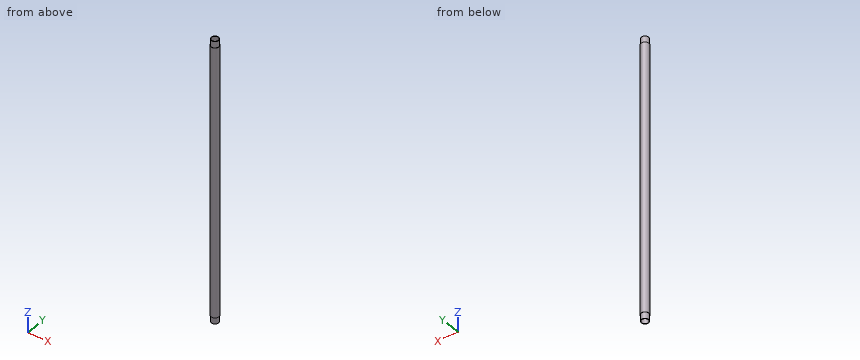
```python
from build123d import *

# Parameters (mm, degrees)
SKETCH2_R           = 6.35
SKETCH2_R_2         = 5.334
BOSS_EXTRUDE1_DEPTH = 457.2


with BuildPart() as part:
    # Sketch2 → Boss-Extrude1 (new body)
    with BuildSketch(Plane.XY):
        Circle(SKETCH2_R)
        Circle(SKETCH2_R_2, mode=Mode.SUBTRACT)
    extrude(amount=BOSS_EXTRUDE1_DEPTH)

    # Sketch3 → Cut-Revolve3 (revolve, cut)
    with BuildSketch(Plane(origin=(0, 0, 0), x_dir=(0, 0, -1), z_dir=(1, 0, 0)), mode=Mode.PRIVATE) as cut_revolve3_sk:
        Polygon((-457.2, 8.954277603), (-457.2, 5.869613211), (-447.050584192, 6.020223087), (-447.050584192, 8.954277603), align=None)
        Polygon((-10.149415808, 8.954277603), (0, 8.954277603), (0, 5.869613211), (-10.149415808, 6.020223087), align=None)
    revolve(cut_revolve3_sk.sketch.rotate(Axis((0, 0, 0), (0, 0, 1)), 90), axis=Axis((0, 0, 0), (0, 0, 1)), mode=Mode.SUBTRACT)


solid = part.part
```
CAD build for the part. Positions are in the model's coordinates, mm. Round coordinates to 2 decimals unless told otherwise and drop trailing zeros. Write each loop counter-clockwise with the first axis right and the second up, starting at its lowest first coordinate (ties: lowest second). Pieces come first, ordered by that corner, then holes.
Item 1: Drop flat-ended pins along their axis: pin 1 Ø6 at (x, z) = (-5, 390.5) entering from -Y; pin 2 Ø2 at (x, z) = (-4.5, 104) entering from -Y; pin 3 Ø6.5 at (x, y) = (-2.5, 0.5) entering from +Z; pin 4 Ø1 at (y, z) = (4.5, 305) entering from +X. Give the stop position or say it passes through.
Filled in:
pin 1: stops at y = -6.03
pin 2: stops at y = -5.3
pin 3: stops at z = 457.2
pin 4: stops at x = 4.93
Item 2: Band-saw the part on A-A on z = 422.5. Write the cut outline in (x, y).
Filled in:
outline: circle Ø12.7 at (0, 0); hole circle Ø10.67 at (0, 0)
Item 3: Drill centre lines: L1, parallel to Y at x = 0, z = 303.5; L2, parallel to X at y = -0.5, z = 99; L3, parallel to Y at x = 4, z = 95.5. Where is each one in solid material? Low to high.
Filled in:
L1: y = -6.35 to -5.33, 5.33 to 6.35
L2: x = -6.33 to -5.31, 5.31 to 6.33
L3: y = -4.93 to -3.53, 3.53 to 4.93
